For this review, use the dimensioned drawing (mm, ordinates from the lowest corner) and the shaded views. A direction names the side the tool comes from. Coordinates: 2 decimals unless noted, no trailing zeros. Loops run counter-clockwise (first coordinate to the right, second up) from the corner with the lowest first, then second, coordinate; pieces in that order, holes last. Notation, with made-up numbers: (62.25, -30) - (73.25, -30) arc R21 ccw to (73.25, -25) - close; hole circle Ø4 at (69, 2.5). An arc over 180 degrees is marked (long way). Use one line per item in the form item = value. Start each with the question number.
(1) For L1, parallel to Y at x = 5, z = 15.5; L2, parallel to Z at x = 4.5, y = 1.75; L3, parallel to X at y = 7.5, z = 27.5 (1 decimal), list the stretches that pass through material, from the lowest coordinate up.
(2) Tool access review of the marked faces 1, 2 and 3: name each direction out of +Z, -Z, +X, -X, +Y, -Y from which nothing blocks a thin tool from reaching the whole face with its end or side.
(3) Add section B-B (z = 7.5). State the section outline as (x, y) points.
(4) Add section C-C (x = 9.5). State the section outline as (y, z) points.
(5) Add section A-A (y = 5.1). State the section outline as (x, z) points (1 decimal).
(6) Clearance check with flat-ended pins moving along their axes: pin 1 Ø5 at (y, z) = (8, 26.5) entering from +X; pin 2 Ø1.4 at (y, z) = (4.5, 29.5) entering from -X; pin 3 Ø6 at (y, z) = (3, 6.5) entering from -X; pin 4 Ø1.5 at (y, z) = (6, 23.5) entering from +X. State where each tip first meets the part, or that it passes through.
(7) The part is to be moulded in two halves that separate along X. For the marked faces 4, 5 and 6, say which applies: pulls with the +X half, pulls with the -X half, needs draft (parallel to the pull), parting line crosses it, or undercut.
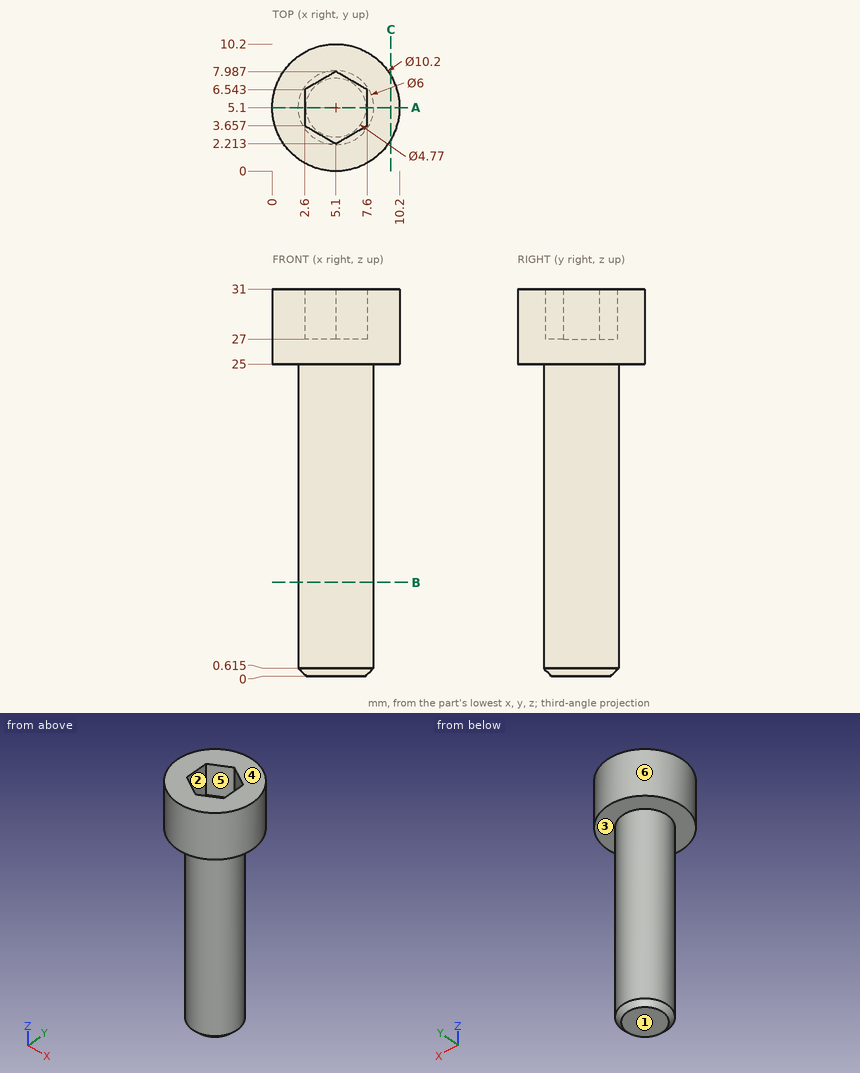
Computed values:
q1.L1 = 2.1 to 8.1
q1.L2 = 25 to 31
q1.L3 = 0.6 to 4.3, 5.9 to 9.6
q2.face_1 = -Z, +X, -X, +Y, -Y
q2.face_2 = +Z
q2.face_3 = -Z
q3.outline = circle Ø6 at (5.1, 5.1)
q4.outline = (2.52, 25) - (7.68, 25) - (7.68, 31) - (2.52, 31) - close
q5.outline = (0, 25) - (2.1, 25) - (2.1, 0.6) - (2.7, 0) - (7.5, 0) - (8.1, 0.6) - (8.1, 25) - (10.2, 25) - (10.2, 31) - (7.6, 31) - (7.6, 27) - (2.6, 27) - (2.6, 31) - (0, 31) - close
q6.pin_1 = 10.18
q6.pin_2 = 0
q6.pin_3 = 2.1
q6.pin_4 = 8.1
q7.face_4 = needs draft
q7.face_5 = undercut
q7.face_6 = parting line crosses it
